Read the model definition and answer for the solid it produces. Units are mm, in the model's axes. Coordinates: 2 decimals unless noted, no trailing zeros. Loops run counter-clockwise (first coordinate to the right, second up) from the corner with the lowest first, then second, coordinate; pieces in that order, holes last. Notation, with made-up numbers: (89, 59) -> (143, 59) arc R12 cw to (143, 80) -> close; hole circle Ø1 at (-19, 43). An arc over 180 degrees is marked (long way). Answer as a JSON object with one key per item and string values. Group by question number.
1) Consider probe 1 along Y at (x, z) = (0, 0.7); probe 2 along Y at (x, z) = (-4.5, -4.75); probe 3 along X at (y, z) = (6.5, -2.5). Determine where each line is inside the solid, lowest interval first. Write a range as [from, to].
2) Section D-D, the plane z = -4.25 is taken. Give the vertices of the cut face in (x, y).
3) Section C-C, the plane z = 1 is taken. Give the vertices of the cut face in (x, y).
4) Section A-A, the plane y = 0 is taken. Give the vertices of the cut face in (x, z).
5) Flat-ended cylindrical pins translate along their axes: P1, Ø12, axis at x = 16, z = -1, coming from the -Y side; P2, Ø12, axis at x = 28.5, z = -2.5, coming from the +Y side; P3, Ø2, axis at x = -21, z = 9.5, coming from the -Y side. Find the tip coordinate at first contact, or state that the pin passes through.
from build123d import *

# Parameters (mm, degrees)
F0_R     = 50
F1_DEPTH = 12.5
F2_R     = 25
F3_DEPTH = 25
F4_R     = 10


with BuildPart() as f1:
    # F0 (on Top) → F1 (new body, symmetric)
    with BuildSketch(Plane.XY):
        Circle(F0_R)
    extrude(amount=F1_DEPTH, both=True)

    # F2 (on face) → F3 (cut)
    with BuildSketch(Plane.XY.offset(12.5)):
        Circle(F2_R)
    extrude(amount=-F3_DEPTH, mode=Mode.SUBTRACT)

    # F4
    f4_edges = [f1.edges().sort_by_distance(p)[0] for p in [
        (-50, 0, 12.5),
        (-50, 0, -12.5),
        (-25, 0, 12.5),
        (-25, 0, -12.5),
    ]]
    fillet(f4_edges, radius=F4_R)


solid = f1.part
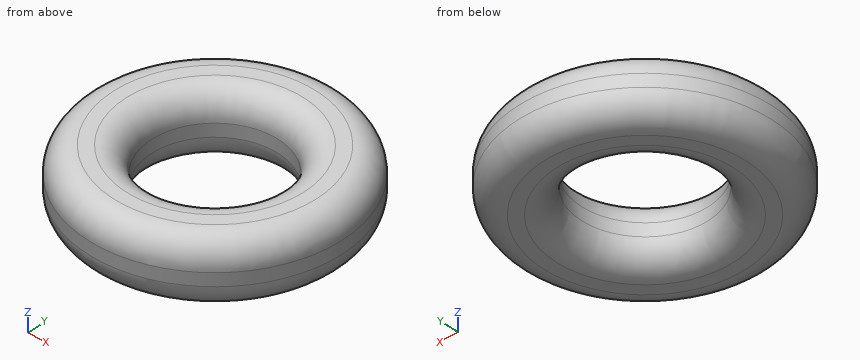
Determined:
{
 "1": {"probe 1": "[-50, -25], [25, 50]", "probe 2": "[-49.54, -24.85], [24.85, 49.54]", "probe 3": "[-49.58, -24.14], [24.14, 49.58]"},
 "2": {"outline": "circle Ø99.69 at (0, 0); hole circle Ø50.31 at (0, 0)"},
 "3": {"outline": "circle Ø100 at (0, 0); hole circle Ø50 at (0, 0)"},
 "4": {"outline": "(-50, -2.5) arc R10 ccw to (-40, -12.5) -> (-35, -12.5) arc R10 ccw to (-25, -2.5) -> (-25, 2.5) arc R10 ccw to (-35, 12.5) -> (-40, 12.5) arc R10 ccw to (-50, 2.5) -> close; (25, -2.5) arc R10 ccw to (35, -12.5) -> (40, -12.5) arc R10 ccw to (50, -2.5) -> (50, 2.5) arc R10 ccw to (40, 12.5) -> (35, 12.5) arc R10 ccw to (25, 2.5) -> close"},
 "5": {"P1": "y = -48.99", "P2": "y = 44.65", "P3": "y = -43.29"}
}
